Design review of the part shown in the three views and the two pictorial views. Dimensions are in mm from the part's minimum x, y and z. A direction names the side the tool comes from. Give positions to 0.01 mm unless a question says otherwise; leave off trailing zeros. Loops run counter-clockwise (first coordinate to the right, second up) from the corner with the lowest first, then second, coordinate; pieces in that order, holes last.
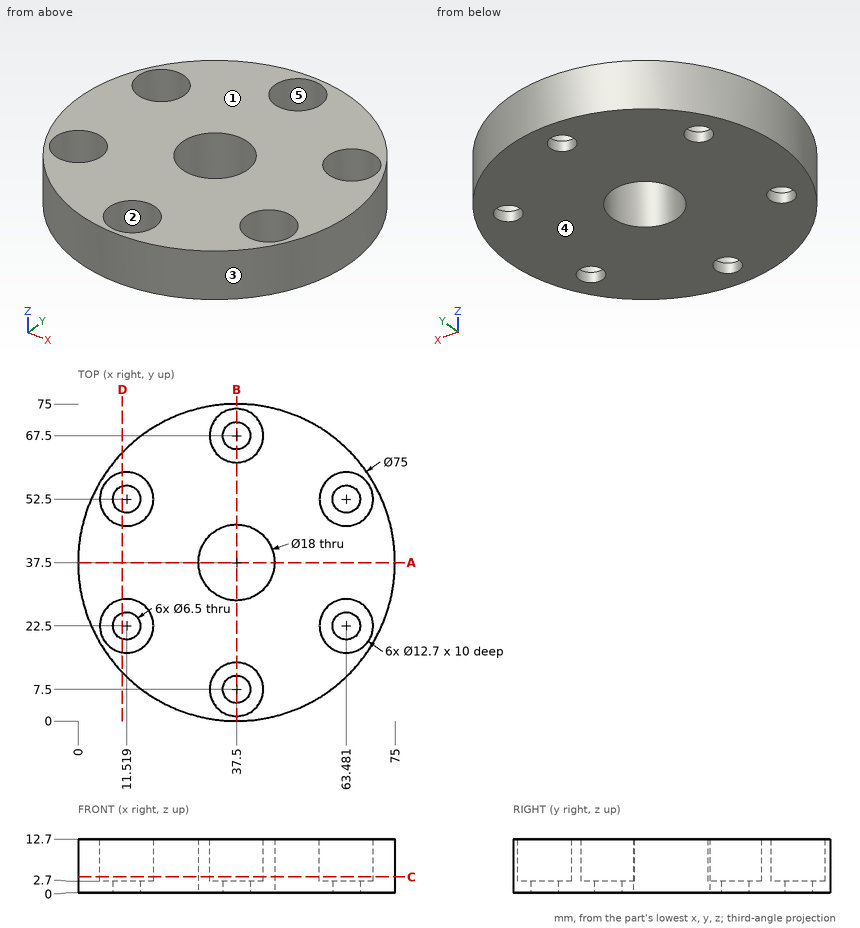
Q1. Consider section C-C on z = 3.75. Give the boundary of the cut face in (x, y).
Answers:
outline: circle Ø75 at (37.5, 37.5); hole circle Ø12.7 at (11.52, 22.5); hole circle Ø12.7 at (11.52, 52.5); hole circle Ø18 at (37.5, 37.5); hole circle Ø12.7 at (37.5, 7.5); hole circle Ø12.7 at (37.5, 67.5); hole circle Ø12.7 at (63.48, 22.5); hole circle Ø12.7 at (63.48, 52.5)
Q2. For pin 1 Ø6.5 at (x, y) = (66, 52.5) entering from +Z; pin 2 Ø1 at (x, y) = (13.5, 11) entering from -Z; pin 3 Ø1.5 at (y, z) = (48, 1.5) entering from -X; pin 4 Ø2 at (y, z) = (53.5, 6.5) entering from -X, all flat-tipped, find the tip position at first contact; note any pin that passes through.
Answers:
pin 1: stops at z = 2.7
pin 2: stops at z = 0
pin 3: stops at x = 1.29
pin 4: stops at x = 3.13
Q3. Consider section B-B on x = 37.5. Give the boundary of the cut face in (y, z).
Answers:
outline: (0, 0) - (4.25, 0) - (4.25, 2.7) - (1.15, 2.7) - (1.15, 12.7) - (0, 12.7) - close; (10.75, 0) - (28.5, 0) - (28.5, 12.7) - (13.85, 12.7) - (13.85, 2.7) - (10.75, 2.7) - close; (46.5, 0) - (64.25, 0) - (64.25, 2.7) - (61.15, 2.7) - (61.15, 12.7) - (46.5, 12.7) - close; (70.75, 0) - (75, 0) - (75, 12.7) - (73.85, 12.7) - (73.85, 2.7) - (70.75, 2.7) - close
Q4. Machinability: for the marked faces 1 and 2, which of the approach directions +Z, -Z, +X, -X, +Y, -Y give a long, thin tool a straight path to every point of the face, cutting with its end or side? Answer none if there is none.
Answers:
face 1: +Z, +X, -X, +Y, -Y
face 2: +Z
Q5. Mouldability with a two-part tool opening along X and no side actions: class the marked faces 3, 4 and 5 as +X half, -X half, draft (parallel to the pull), parting line (faces both ways), or undercut.
Answers:
face 3: parting line
face 4: draft
face 5: undercut
Q6. Consider section A-A on y = 37.5. Give the boundary of the cut face in (x, z), plus the area to 3 significant figures.
Answers:
outline: (0, 0) - (28.5, 0) - (28.5, 12.7) - (0, 12.7) - close; (46.5, 0) - (75, 0) - (75, 12.7) - (46.5, 12.7) - close
area: 724 mm2
Q7. For probe 1 along Y at (x, z) = (37.5, 0.6); probe 2 along Y at (x, z) = (37.5, 9.75); probe 3 along X at (y, z) = (56, 10.5), list the stretches that pass through material, from the lowest coordinate up.
Answers:
probe 1: y = 0 to 4.25, 10.75 to 28.5, 46.5 to 64.25, 70.75 to 75
probe 2: y = 0 to 1.15, 13.85 to 28.5, 46.5 to 61.15, 73.85 to 75
probe 3: x = 4.88 to 6.22, 16.82 to 58.18, 68.78 to 70.12
Q8. Consider section D-D on x = 10.5. Give the boundary of the cut face in (y, z).
Answers:
outline: (11.48, 0) - (19.41, 0) - (19.41, 2.7) - (16.23, 2.7) - (16.23, 12.7) - (11.48, 12.7) - close; (25.59, 0) - (49.41, 0) - (49.41, 2.7) - (46.23, 2.7) - (46.23, 12.7) - (28.77, 12.7) - (28.77, 2.7) - (25.59, 2.7) - close; (55.59, 0) - (63.52, 0) - (63.52, 12.7) - (58.77, 12.7) - (58.77, 2.7) - (55.59, 2.7) - close
